from build123d import *

# Parameters (mm, degrees)
F0_W     = 76.2
F0_H     = 76.2
F1_DEPTH = 76.2
F2_W     = 25.4
F2_H     = 25.4
F3_DEPTH = 25.4
F5_D     = 25.4


# Not quite as in the source:
# - the program builds the solid bodies; features that only make, move or delete a surface that nothing else refers to are left out


with BuildPart() as f1:
    # F0 (on Front) → F1 (new body)
    with BuildSketch(Plane.XZ):
        with Locations((38.1, 38.1)):
            Rectangle(F0_W, F0_H)
    extrude(amount=F1_DEPTH)

    # F2 (on face) → F3 (join)
    with BuildSketch(Plane.XZ.offset(76.2)):
        with Locations((38.1, 38.1)):
            Rectangle(F2_W, F2_H)
    extrude(amount=F3_DEPTH)

    # F5 (through all)
    with Locations(Plane.XY.offset(76.2)):
        with Locations((38.1, -38.1)):
            Hole(F5_D / 2)


solid = f1.part
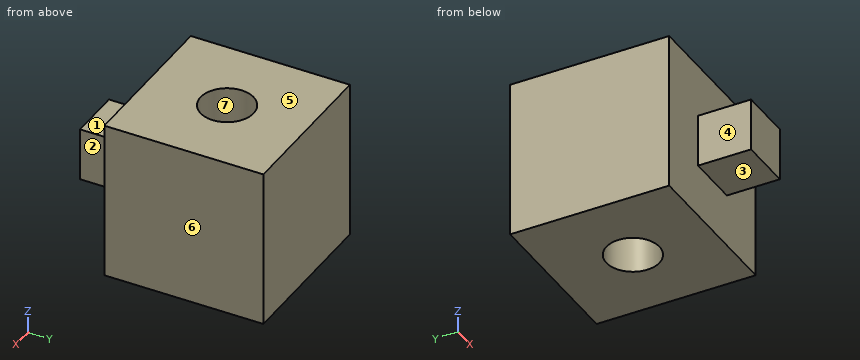
Could you check a few things on this model? Use its own coordinates, in mm. Face numbers are marked on the shaded views. A direction names the side the tool comes from. Give positions to 0.01 mm unless a question says otherwise; leave off trailing zeros. Order: outer loops, then holes, each group sorted by start corner. A loop starts at its lowest first (then second) coordinate and runs counter-clockwise, first axis right, second up. Notation, with made-up numbers: (-40, 19.5) -> (9, 19.5) arc R16 cw to (9, 39.5) -> close; hole circle Ø1 at (55.5, -15.5). An arc over 180 degrees is marked (long way). Answer in a Markdown table with one row per item. Add a question column.
Item 1: Imagine slicing it at B-B (y = -38.1). List the corners of the cut face in (x, z) for me, and give its area (3 significant figures).
Item 2: Imagine slicing it at C-C (x = 38.1). List the corners of the cut face in (y, z) for me, and give its area (3 significant figures).
Item 3: We'd pull the mould along X, two halves only. Please class the marked faces 5, 6 and 7: pulls with the +X half, pulls with the -X half, needs draft (parallel to the pull), parting line crosses it, or undercut.
Item 4: I'm going to push flat-ended pins straight in: P1, Ø6, axis at x = 64, z = 33, coming from the -Y side; P2, Ø12.5, axis at y = -86, z = 39, coming from the -X side. Where does each tip first touch, or does it pass through?
Item 5: Imagine slicing it at A-A (z = 45). List the corners of the cut face in (x, y) for me, and give its area (3 significant figures).
Item 6: Please list where these lines run through material, in increasing order: probe 1 along X at (y, z) = (-38, 44); probe 2 along Y at (x, z) = (38.1, 35.5); probe 3 along Y at (x, z) = (60, 32).
Item 7: Imagine slicing it at D-D (z = 12). List the corners of the cut face in (x, y) for me, and give its area (3 significant figures).
Item 8: For the marked faces 1, 2, 3 and 4, which set-ups out of +Z, -Z, +X, -X, +Y, -Y let a thin tool reach every point of the face, with its end or its side?
Result:
| question | item | result |
|---|---|---|
| 1 | outline | (0, 0) -> (25.4, 0) -> (25.4, 76.2) -> (0, 76.2) -> close; (50.8, 0) -> (76.2, 0) -> (76.2, 76.2) -> (50.8, 76.2) -> close |
| 1 | area | 3,870 mm2 |
| 2 | outline | (-101.6, 25.4) -> (-76.2, 25.4) -> (-76.2, 0) -> (-50.8, 0) -> (-50.8, 76.2) -> (-76.2, 76.2) -> (-76.2, 50.8) -> (-101.6, 50.8) -> close; (-25.4, 0) -> (0, 0) -> (0, 76.2) -> (-25.4, 76.2) -> close |
| 2 | area | 4,520 mm2 |
| 3 | face 5 | needs draft |
| 3 | face 6 | pulls with the +X half |
| 3 | face 7 | undercut |
| 4 | P1 | y = -76.2 |
| 4 | P2 | x = 25.4 |
| 5 | outline | (0, -76.2) -> (25.4, -76.2) -> (25.4, -101.6) -> (50.8, -101.6) -> (50.8, -76.2) -> (76.2, -76.2) -> (76.2, 0) -> (0, 0) -> close; hole circle Ø25.4 at (38.1, -38.1) |
| 5 | area | 5,940 mm2 |
| 6 | probe 1 | 0 to 25.4, 50.8 to 76.2 |
| 6 | probe 2 | -101.6 to -50.8, -25.4 to 0 |
| 6 | probe 3 | -76.2 to 0 |
| 7 | outline | (0, -76.2) -> (76.2, -76.2) -> (76.2, 0) -> (0, 0) -> close; hole circle Ø25.4 at (38.1, -38.1) |
| 7 | area | 5,300 mm2 |
| 8 | face 1 | +Z, +X, -X, -Y |
| 8 | face 2 | +Z, -Z, +X, -Y |
| 8 | face 3 | -Z, +X, -X, -Y |
| 8 | face 4 | +Z, -Z, -X, -Y |
